from build123d import *

# Parameters (mm, degrees)
SKETCH2_W           = 110
SKETCH2_H           = 40
BOSS_EXTRUDE1_DEPTH = 100
SKETCH3_W           = 30
SKETCH3_H           = 20
CUT_EXTRUDE1_DEPTH  = 100
SKETCH4_W           = 20
SKETCH4_H           = 100
BOSS_EXTRUDE3_DEPTH = 50
CUT_EXTRUDE2_DEPTH  = 50
SKETCH7_W           = 40
SKETCH7_H           = 20
BOSS_EXTRUDE4_DEPTH = 30
CUT_EXTRUDE3_DEPTH  = 30
SKETCH9_W           = 50
SKETCH9_H           = 50
BOSS_EXTRUDE5_DEPTH = 20
CUT_EXTRUDE5_DEPTH  = 20
CUT_EXTRUDE6_DEPTH  = 20


with BuildPart() as part:
    # Sketch2 → Boss-Extrude1 (new body)
    with BuildSketch(Plane.XY):
        with Locations((55, 20)):
            Rectangle(SKETCH2_W, SKETCH2_H)
    extrude(amount=BOSS_EXTRUDE1_DEPTH)

    # Sketch3 → Cut-Extrude1 (cut)
    with BuildSketch(Plane.XY.offset(100)):
        with Locations((75, 30)):
            Rectangle(SKETCH3_W, SKETCH3_H)
        with Locations((15, 30)):
            Rectangle(SKETCH3_W, SKETCH3_H)
    extrude(amount=-CUT_EXTRUDE1_DEPTH, mode=Mode.SUBTRACT)

    # Sketch4 → Boss-Extrude3 (add)
    with BuildSketch(Plane(origin=(0, 0, 0), x_dir=(-1, 0, 0), z_dir=(0, -1, 0))):
        with Locations((-100, -50)):
            Rectangle(SKETCH4_W, SKETCH4_H)
    extrude(amount=BOSS_EXTRUDE3_DEPTH)

    # Sketch6 → Cut-Extrude2 (cut)
    with BuildSketch(Plane.ZY.offset(-90)):
        with BuildLine():
            Line((80, -30), (80, -50))
            Line((80, -50), (100, -50))
            Line((100, -50), (100, -10))
            ThreePointArc((100, -10), (85.857864376, -15.857864376), (80, -30))
        make_face()
        with BuildLine():
            Line((20, -30), (20, -50))
            Line((20, -50), (0, -50))
            Line((0, -50), (0, -10))
            ThreePointArc((0, -10), (14.142135624, -15.857864376), (20, -30))
        make_face()
    extrude(amount=-CUT_EXTRUDE2_DEPTH, mode=Mode.SUBTRACT)

    # Sketch7 → Boss-Extrude4 (add)
    with BuildSketch(Plane(origin=(0, 0, 0), x_dir=(-1, 0, 0), z_dir=(0, -1, 0))):
        with Locations((-70, -50)):
            Rectangle(SKETCH7_W, SKETCH7_H)
    extrude(amount=BOSS_EXTRUDE4_DEPTH)

    # Sketch8 → Cut-Extrude3 (cut)
    with BuildSketch(Plane.XY.offset(60)):
        Polygon((90, -30), (50, 0), (50, -30), align=None)
    extrude(amount=-CUT_EXTRUDE3_DEPTH, mode=Mode.SUBTRACT)

    # Sketch9 → Boss-Extrude5 (add)
    with BuildSketch(Plane(origin=(0, 0, 0), x_dir=(-1, 0, 0), z_dir=(0, -1, 0))):
        with Locations((25, -25)):
            Rectangle(SKETCH9_W, SKETCH9_H)
    extrude(amount=-BOSS_EXTRUDE5_DEPTH)

    # Sketch10 → Cut-Extrude5 (cut)
    with BuildSketch(Plane(origin=(0, 0, 0), x_dir=(-1, 0, 0), z_dir=(0, -1, 0))):
        with BuildLine():
            Line((30, -50), (0, -50))
            Line((0, -50), (0, -80))
            ThreePointArc((0, -80), (-21.213203436, -28.786796564), (30, -50))
        make_face()
    extrude(amount=-CUT_EXTRUDE5_DEPTH, mode=Mode.SUBTRACT)

    # Sketch12 → Cut-Extrude6 (cut)
    with BuildSketch(Plane(origin=(0, 0, 0), x_dir=(-1, 0, 0), z_dir=(0, -1, 0))):
        with BuildLine():
            Line((50, -50), (50, 0))
            Line((50, 0), (0, 0))
            ThreePointArc((0, 0), (35.355339059, -14.644660941), (50, -50))
        make_face()
    extrude(amount=-CUT_EXTRUDE6_DEPTH, mode=Mode.SUBTRACT)


solid = part.part
Can you work these out from the model? Positions are in its coordinate system, mm. A direction names the side the tool comes from. Give positions to 0.01 mm unless a question says otherwise; leave off trailing zeros. Loops run counter-clockwise (first coordinate to the right, second up) from the corner with the lowest first, then second, coordinate; pieces in that order, holes last. Notation, with made-up numbers: (41, 60.5) - (91, 60.5) arc R35 cw to (91, 94.5) - close; hole circle Ø1 at (85.25, 53). An arc over 180 degrees is marked (long way). Return JSON: item names as keys, results as strings.
1. I want a section at A-A on y = 34. Please give me the cut outline in (x, z), and give its area (3 significant figures).
Output values:
{"outline": "(30, 0) - (60, 0) - (60, 100) - (30, 100) - close; (90, 0) - (110, 0) - (110, 100) - (90, 100) - close", "area": "5,000 mm²"}
2. If I drill on line 1 (X direction, y = 27.5, z = 17.5); line 2 (Y direction, x = 75.5, z = 23.5); line 3 (Y direction, x = 31, z = 38.5), over which ranges is the centre line in solid material (lowest first)?
Output values:
{"line 1": "x = 30 to 60, 90 to 110", "line 2": "y = 0 to 20", "line 3": "y = 0 to 40"}
3. We'd pull the mould along X, two halves only. Please class faces 6 (the face through (75, 20, 51)), 7 (the face through (100, -40, 80)), 8 (the face through (90, -30.2, 50.7)): +X half, -X half, draft (parallel to the pull), parting line (faces both ways), or undercut.
Output values:
{"face 6": "undercut", "face 7": "draft", "face 8": "-X half"}
4. I want a section at B-B on z = 32. Please give me the cut outline in (x, y), and give its area (3 significant figures).
Output values:
{"outline": "(-46.65, 0) - (-24, 0) - (-24, 20) - (-46.65, 20) - close; (24, 0) - (90, 0) - (90, -50) - (110, -50) - (110, 40) - (90, 40) - (90, 20) - (60, 20) - (60, 40) - (30, 40) - (30, 20) - (24, 20) - close", "area": "4,170 mm²"}
5. I want a section at C-C on y = 2.5. Please give me the cut outline in (x, z).
Output values:
{"outline": "(-50, 50) arc R50 ccw to (0, 0) - (110, 0) - (110, 100) - (0, 100) - (0, 80) arc R30 cw (long way) to (-30, 50) - close"}
6. I want a section at D-D on z = 91. Please give me the cut outline in (x, y).
Output values:
{"outline": "(0, 0) - (90, 0) - (90, -12.14) - (110, -12.14) - (110, 40) - (90, 40) - (90, 20) - (60, 20) - (60, 40) - (30, 40) - (30, 20) - (0, 20) - close"}
7. I'm going to push flat-ended pins straight in: pin 1 Ø25 at (x, z) = (9.5, 29) entering from +Y; pin 2 Ø6 at (x, y) = (96.5, -42) entering from +Z; pin 3 Ø5 at (x, y) = (-30.5, 0.5) entering from +Z. Where does each tip first touch, or does it pass through?
Output values:
{"pin 1": "stops at y = 20", "pin 2": "stops at z = 80", "pin 3": "stops at z = 50"}
8. For faces 1 (the face through (37, 0, 49)), 2 (the face through (75, -11, 60)), 3 (the face through (60, 30, 51)), 4 (the face through (-9, 20, 19)), 5 (the face through (100, -40, 20)), which set-ups out of +Z, -Z, +X, -X, +Y, -Y let a thin tool reach every point of the face, with its end or its side?
Output values:
{"face 1": "-X, -Y", "face 2": "+Z, -X, -Y", "face 3": "+Z, -Z, +Y", "face 4": "+Z, -Z, -X, +Y", "face 5": "-Z, +X, -X, -Y"}
